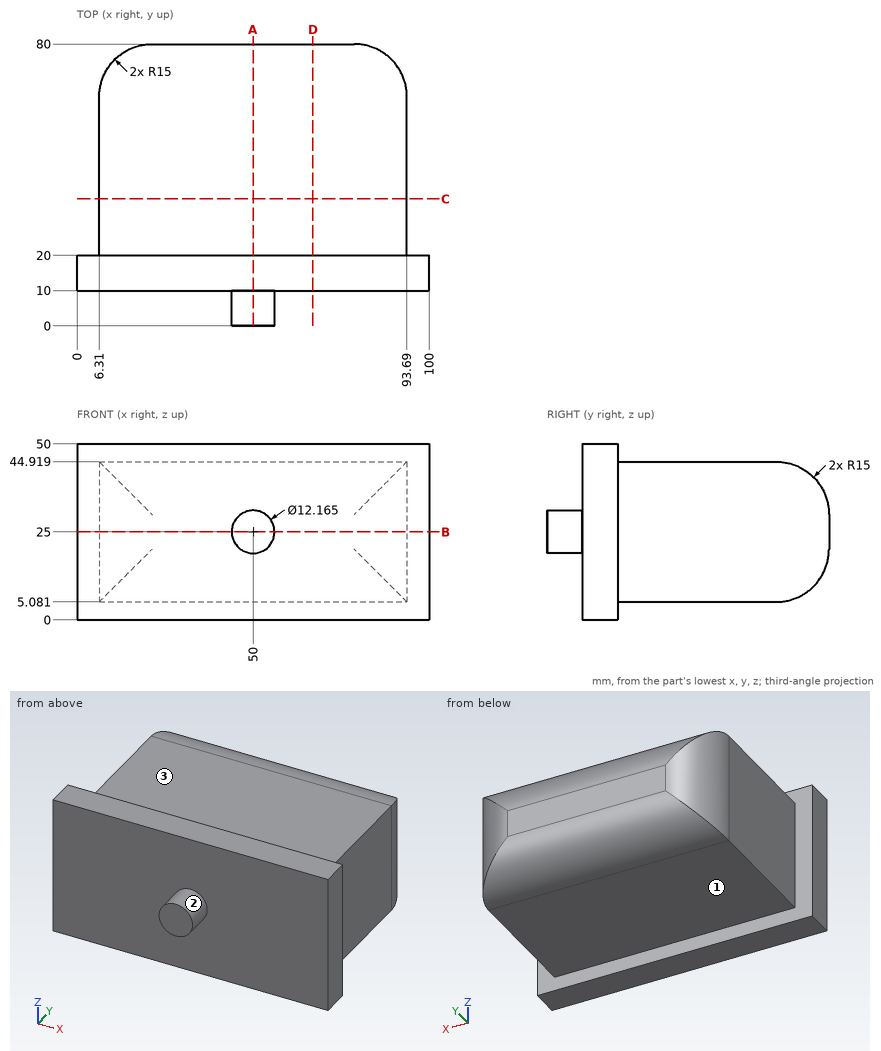
The figure shows three views and two pictorial views of one solid part (mm, origin at its lowest corner). Answer the questions. A direction names the side the tool comes from. Round coordinates to 2 decimals unless told otherwise and drop trailing zeros. Loops run counter-clockwise (first coordinate to the right, second up) from the corner with the lowest first, then second, coordinate; pieces in that order, holes last. Notation, with made-up numbers: (54, -23.5) - (112, -23.5) arc R22 ccw to (112, 0.5) - close; hole circle Ø3 at (34.25, -7). An arc over 180 degrees is marked (long way). One line per question, with ' | ' between items. Start each with the question number.
Q1. Section C-C on y = 36 is taken. Give the vertices of the cut face in (x, z), plus the area to 3 significant figures.
Q2. Section B-B on z = 25 is taken. Give the vertices of the cut face in (x, y).
Q3. Section D-D on x = 67 is taken. Give the vertices of the cut face in (y, z), plus the area to 3 significant figures.
Q4. Flat-ended cylindrical pins translate along their axes: pin 1 (8 mm diameter, centred on x = 30, y = 68, fed in from -Z); pin 2 (6 mm diameter, centred on y = 65.5, z = 38.5, fed in from +X); pin 3 (6 mm diameter, centred on x = 23, y = 58, fed in from +Z). Find the tip coordinate at first contact, or state that the pin passes through.
Q5. Section A-A on x = 50 is taken. Give the vertices of the cut face in (y, z), plus the area to 3 significant figures.
Q6. For the marked faces 1, 2 and 3, determine the directions among +Z, -Z, +X, -X, +Y, -Y from which every point of the face is accessible in a straight line to the end or side of a thin tool.
Q7. Find the intervals of material crossed by L1, parallel to X at y = 33, z = 20; L2, parallel to Y at x = 60.5, z = 26; L3, parallel to Z at x = 81, y = 40.5, in increasing order.
Established:
1) outline: (6.31, 5.08) - (93.69, 5.08) - (93.69, 44.92) - (6.31, 44.92) - close | area: 3,480 mm²
2) outline: (0, 10) - (43.92, 10) - (43.92, 0) - (56.08, 0) - (56.08, 10) - (100, 10) - (100, 20) - (93.69, 20) - (93.69, 65) arc R15 ccw to (78.69, 80) - (21.31, 80) arc R15 ccw to (6.31, 65) - (6.31, 20) - (0, 20) - close
3) outline: (10, 0) - (20, 0) - (20, 5.08) - (65, 5.08) arc R15 ccw to (80, 20.08) - (80, 29.92) arc R15 ccw to (65, 44.92) - (20, 44.92) - (20, 50) - (10, 50) - close | area: 2,790 mm²
4) pin 1: z = 5.08 | pin 2: x = 93.69 | pin 3: z = 44.92
5) outline: (0, 18.92) - (10, 18.92) - (10, 0) - (20, 0) - (20, 5.08) - (65, 5.08) arc R15 ccw to (80, 20.08) - (80, 29.92) arc R15 ccw to (65, 44.92) - (20, 44.92) - (20, 50) - (10, 50) - (10, 31.08) - (0, 31.08) - close | area: 2,920 mm²
6) face 1: -Z, +X, -X, +Y | face 2: -Y | face 3: +Z, +X, -X, +Y
7) L1: 6.31 to 93.69 | L2: 10 to 80 | L3: 5.08 to 44.92
